The listing builds one solid part. Answer for the finished solid, in the listing's coordinates (mm). A direction names the side the tool comes from. Coordinates: 2 decimals unless noted, no trailing zeros. Order: outer loops, then holes, each group sorted by start corner. A loop starts at its lowest first (then second) coordinate and runs counter-clockwise, first axis right, second up. Notation, with made-up numbers: (53.25, 47) -> (78.25, 47) arc R30 ccw to (78.25, 83) -> close; hole circle Ø11 at (13.5, 88). An arc over 180 degrees is marked (long way). One line per question, with ' | ' between items.
from build123d import *

# Parameters (mm, degrees)
BOSS_EXTRUDE1_DEPTH   = 10
BOSS_EXTRUDE1_2_DEPTH = 10
BOSS_EXTRUDE1_3_DEPTH = 10
BOSS_EXTRUDE1_4_DEPTH = 10
SKETCH1_W             = 20
SKETCH1_H             = 5
BOSS_EXTRUDE1_5_DEPTH = 10
BOSS_EXTRUDE1_6_DEPTH = 10
SKETCH2_R             = 50
BOSS_EXTRUDE2_DEPTH   = 5
SKETCH3_R             = 1.525
CUT_EXTRUDE1_DEPTH    = 30
SKETCH4_R             = 1.525
CUT_EXTRUDE2_DEPTH    = 30
SKETCH5_R             = 1.525
CUT_EXTRUDE3_DEPTH    = 30


with BuildPart() as part:
    # Sketch1 → Boss-Extrude1 (new body)
    with BuildSketch(Plane(origin=(0, 0, 0), x_dir=(1, 0, 0), z_dir=(0, 1, 0))):
        Polygon((44.174682453, 101.512794416), (34.174682453, 84.192286341), (38.504809472, 81.692286341), (48.504809472, 99.012794416), align=None)
    extrude(amount=BOSS_EXTRUDE1_DEPTH)



with BuildPart() as body_2:
    # Sketch1 → Boss-Extrude1 2 (new body)
    with BuildSketch(Plane(origin=(0, 0, 0), x_dir=(1, 0, 0), z_dir=(0, 1, 0))):
        Polygon((61.495190528, 91.512794416), (65.825317547, 89.012794416), (55.825317547, 71.692286341), (51.495190528, 74.192286341), align=None)
    extrude(amount=BOSS_EXTRUDE1_2_DEPTH)


with BuildPart() as body_3:
    # Sketch1 → Boss-Extrude1 3 (new body)
    with BuildSketch(Plane(origin=(0, 0, 0), x_dir=(1, 0, 0), z_dir=(0, 1, 0))):
        Polygon((65.825317547, -89.012794416), (55.825317547, -71.692286341), (51.495190528, -74.192286341), (61.495190528, -91.512794416), align=None)
    extrude(amount=BOSS_EXTRUDE1_3_DEPTH)


with BuildPart() as body_4:
    # Sketch1 → Boss-Extrude1 4 (new body)
    with BuildSketch(Plane(origin=(0, 0, 0), x_dir=(1, 0, 0), z_dir=(0, 1, 0))):
        Polygon((48.504809472, -99.012794416), (44.174682453, -101.512794416), (34.174682453, -84.192286341), (38.504809472, -81.692286341), align=None)
    extrude(amount=BOSS_EXTRUDE1_4_DEPTH)


with BuildPart() as body_5:
    # Sketch1 → Boss-Extrude1 5 (new body)
    with BuildSketch(Plane(origin=(0, 0, 0), x_dir=(1, 0, 0), z_dir=(0, 1, 0))):
        with Locations((-100, -10)):
            Rectangle(SKETCH1_W, SKETCH1_H)
    extrude(amount=BOSS_EXTRUDE1_5_DEPTH)


with BuildPart() as body_6:
    # Sketch1 → Boss-Extrude1 6 (new body)
    with BuildSketch(Plane(origin=(0, 0, 0), x_dir=(1, 0, 0), z_dir=(0, 1, 0))):
        with Locations((-100, 10)):
            Rectangle(SKETCH1_W, SKETCH1_H)
    extrude(amount=BOSS_EXTRUDE1_6_DEPTH)


with BuildPart() as part_1:
    add(part.part)

    add(body_2.part)  # Boss-Extrude2 merges body 2

    add(body_3.part)  # Boss-Extrude2 merges body 3

    add(body_4.part)  # Boss-Extrude2 merges body 4

    add(body_5.part)  # Boss-Extrude2 merges body 5

    add(body_6.part)  # Boss-Extrude2 merges body 6
    # Sketch2 → Boss-Extrude2 (add)
    with BuildSketch(Plane(origin=(0, 0, 0), x_dir=(1, 0, 0), z_dir=(0, 1, 0))):
        Polygon((-117, 107), (-107, 117), (107, 117), (117, 107), (117, -107), (107, -117), (-107, -117), (-117, -107), align=None)
        with Locations(Location((0, 0, 0), (0, 0, 270))):
            Circle(SKETCH2_R, mode=Mode.SUBTRACT)
    extrude(amount=-BOSS_EXTRUDE2_DEPTH)

    # Sketch3 → Cut-Extrude1 (cut)
    with BuildSketch(Plane.XY.offset(12.5)):
        with Locations((-100, 7)):
            Circle(SKETCH3_R)
    extrude(amount=-CUT_EXTRUDE1_DEPTH, mode=Mode.SUBTRACT)

    # Sketch4 → Cut-Extrude2 (cut)
    with BuildSketch(Plane(origin=(10.825317547, 0, -6.25), x_dir=(-0.5000000000000004, 0, -0.8660254037844385), z_dir=(0.8660254037844384, 0, -0.5000000000000003))):
        with Locations((-100, 7)):
            Circle(SKETCH4_R)
    extrude(amount=-CUT_EXTRUDE2_DEPTH, mode=Mode.SUBTRACT)

    # Sketch5 → Cut-Extrude3 (cut)
    with BuildSketch(Plane(origin=(-10.825317547, 0, -6.25), x_dir=(-0.5000000000000001, 0, 0.8660254037844386), z_dir=(-0.8660254037844386, 0, -0.5000000000000001))):
        with Locations((-100, 7)):
            Circle(SKETCH5_R)
    extrude(amount=-CUT_EXTRUDE3_DEPTH, mode=Mode.SUBTRACT)


solid = part_1.part
Item 1: For faces 4 (the face through (-110, 5, 10)), 5 (the face through (-100, 5, 7.5)), 6 (the face through (-100, 5, 12.5)), determine the directions among +Z, -Z, +X, -X, +Y, -Y from which every point of the face is accessible in a straight line to the end or side of a thin tool.
Computed values:
face 4: +Z, -Z, -X, +Y | face 5: +X, -X, +Y | face 6: +Z, +X, -X, +Y
Item 2: Find the intervals of material crossed by L1, parallel to Y at x = -100, z = -9.7 (3 decimals); L2, parallel to Z at x = 60.5, y = 1; L3, parallel to X at y = -2, z = 33, in increasing order.
Computed values:
L1: y = -5 to 5.475, 8.525 to 10 | L2: z = -89.79 to -79.79, 79.79 to 89.79 | L3: x = -117 to -37.56, 37.56 to 117
Item 3: Section B-B, the plane x = 0 is taken. Give the vertices of the cut face in (y, z).
Computed values:
outline: (-5, -117) -> (0, -117) -> (0, -50) -> (-5, -50) -> close; (-5, 50) -> (0, 50) -> (0, 117) -> (-5, 117) -> close
Item 4: Each of these flat-tipped pins is pushed along its axis until it touches: pin 1 Ø8 at (x, y) = (68.5, 8) entering from +Z; pin 2 Ø2.5 at (y, z) = (7, 9.5) entering from +X; pin 3 Ø5 at (y, z) = (8.5, -84.5) entering from -X. Where does it stop, or does it pass through?
Computed values:
pin 1: stops at z = 89.78 | pin 2: stops at x = -90 | pin 3: stops at x = 34.17
Item 5: Section A-A, the plane z = 0 is taken. Give the vertices of the cut face in (x, y), plus the area to 3 significant figures.
Computed values:
outline: (-117, -5) -> (-50, -5) -> (-50, 0) -> (-117, 0) -> close; (50, -5) -> (117, -5) -> (117, 0) -> (50, 0) -> close | area: 670 mm^2
Item 6: Section C-C, the plane x = -85 is taken. Give the vertices of the cut face in (y, z), plus the area to 3 significant figures.
Computed values:
outline: (-5, -117) -> (0, -117) -> (0, 117) -> (-5, 117) -> close | area: 1,170 mm^2
Item 7: Determine the mould class of faces 1 (the face through (-1, -2, -117)), 2 (the face through (60.895, 4.93, -80.474)), 3 (the face through (59, 10, -82)) for opening direction Z: pulls with the +Z half, pulls with the -Z half, needs draft (parallel to the pull), parting line crosses it, or undercut.
Computed values:
face 1: pulls with the -Z half | face 2: undercut | face 3: needs draft
